```python
from build123d import *

# Parameters (mm, degrees)
F0_W      = 78
F0_H      = 80
F1_DEPTH  = 100
F2_T      = -2
F3_W      = 74
F3_H      = 2
F4_DEPTH  = 75
F5_W      = 72.1805748753
F5_H      = 9.0993850976
F6_DEPTH  = 25
F8_DEPTH  = 38.5
F9_W      = 29
F9_H      = 2
F10_DEPTH = 6


with BuildPart() as f1:
    # F0 (on Top) → F1 (new body)
    with BuildSketch(Plane.XY):
        with Locations((39, 40)):
            Rectangle(F0_W, F0_H)
    extrude(amount=F1_DEPTH)

    # F2
    f2_openings = [f1.faces().sort_by_distance(p)[0] for p in [
        (39, 40, 100),
    ]]
    offset(amount=F2_T, openings=f2_openings)

    # F3 (on face) → F4 (join)
    with BuildSketch(Plane.XY.offset(2)):
        with Locations((39, 11.5)):
            Rectangle(F3_W, F3_H)
    extrude(amount=F4_DEPTH)

    # F5 (on face) → F6 (join)
    with BuildSketch(Plane.XY.offset(2)):
        with Locations((39.9097125623, 6.5496925488)):
            Rectangle(F5_W, F5_H)
    extrude(amount=F6_DEPTH)

    # F7 (on face) → F8 (cut)
    with BuildSketch(Plane.XY.offset(27)):
        with BuildLine():
            Line((70.4722125623, 10.5), (9.4722125623, 10.5))
            ThreePointArc((9.4722125623, 10.5), (5.2222125623, 6.25), (9.4722125623, 2))
            Line((9.4722125623, 2), (70.4722125623, 2))
            ThreePointArc((70.4722125623, 2), (74.7222125623, 6.25), (70.4722125623, 10.5))
        make_face()
    extrude(amount=-F8_DEPTH, mode=Mode.SUBTRACT)

    # F9 (on face) → F10 (cut)
    with BuildSketch(Plane.XY.offset(100)):
        with Locations((61.5, 79)):
            Rectangle(F9_W, F9_H)
    extrude(amount=-F10_DEPTH, mode=Mode.SUBTRACT)


solid = f1.part
```
Design review of the part built by this model. Coordinates are the model's own, in mm. A direction names the side the tool comes from. Coordinates: 2 decimals unless noted, no trailing zeros. Order: outer loops, then holes, each group sorted by start corner. A loop starts at its lowest first (then second) coordinate and runs counter-clockwise, first axis right, second up.
1) Take a section at C-C, the plane x = 54. Give the boundary of the cut face in (y, z).
2) Wall thickness on line 1 along Y through (x, z) = (48.5, 37); line 2 along X through (y, z) = (52, 84.5); line 3 along Y through (x, z) = (67, 81.5): over which ranges is each line inside the solid? List them lowest first.
3) Mouldability with a two-part tool opening along Y and no side actions: class faces 1 (the flat face through (38, 80, 49)), 2 (the flat face through (0, 39, 49)), 3 (the flat face through (75, 6, 27)) as +Y half, -Y half, draft (parallel to the pull), parting line (faces both ways), or undercut.
4) For faces 4 (the flat face through (2, 39, 50)), 5 (the cylindrical face through (5.223, 6.343, 13.689)), 6 (the flat face through (38, 41, 0)), list the 3-axis set-ups (+Z, -Z, +X, -X, +Y, -Y) from which the entire face can be reached by the end or side of a thin tool; tool diameter is ignored.
5) Take a section at A-A, the plane y = 6.25. Give the boundary of the cut face in (x, z), and give its area (3 significant figures).
6) Take a section at D-D, the plane y = 62.5. Give the boundary of the cut face in (x, z).
7) Clearance check with flat-ended pins moving along their axes: pin 1 (1.6 mm diameter, centred on x = 66, y = 79.5, fed in from +Z); pin 2 (1.6 mm diameter, centred on x = 52, y = 11, fed in from +Z); pin 3 (0.9 mm diameter, centred on x = 3, y = 6, fed in from +Z). State where each tip first meets the part, or that it passes through.
8) Take a section at B-B, the plane z = 17.5. Give the boundary of the cut face in (x, y), and give its area (3 significant figures).
Returned:
1. outline: (0, 0) - (2, 0) - (2, 100) - (0, 100) - close; (10.5, 0) - (80, 0) - (80, 94) - (78, 94) - (78, 2) - (12.5, 2) - (12.5, 77) - (10.5, 77) - close
2. line 1: y = 0 to 2, 10.5 to 12.5, 78 to 80
2. line 2: x = 0 to 2, 76 to 78
2. line 3: y = 0 to 2, 78 to 80
3. face 1: +Y half
3. face 2: draft
3. face 3: undercut
4. face 4: +Z
4. face 5: +Z, -Z
4. face 6: -Z, +X, -X, +Y, -Y
5. outline: (0, 0) - (5.22, 0) - (5.22, 27) - (3.82, 27) - (3.82, 2) - (2, 2) - (2, 100) - (0, 100) - close; (74.72, 0) - (78, 0) - (78, 100) - (76, 100) - (76, 27) - (74.72, 27) - close
5. area: 476 mm2
6. outline: (0, 0) - (78, 0) - (78, 100) - (76, 100) - (76, 2) - (2, 2) - (2, 100) - (0, 100) - close
7. pin 1: stops at z = 94
7. pin 2: stops at z = 77
7. pin 3: stops at z = 2
8. outline: (0, 0) - (78, 0) - (78, 80) - (0, 80) - close; hole (2, 2) - (3.82, 2) - (3.82, 10.5) - (2, 10.5) - close; hole (2, 12.5) - (76, 12.5) - (76, 78) - (2, 78) - close; hole (9.47, 2) - (70.47, 2) arc R4.25 ccw to (70.47, 10.5) - (9.47, 10.5) arc R4.25 ccw to start
8. area: 802 mm2
